```python
from build123d import *

# Parameters (mm, degrees)
F0_W         = 20
F0_H         = 20
F1_DEPTH     = 20.8070650697
F3_DEPTH     = 10
F4_T4_DEPTH  = 23.6433897602
F4_T10_DEPTH = 23.6433897602
F4_T15_DEPTH = 23.6433897602
F4_T20_DEPTH = 23.6433897602
F4_T26_DEPTH = 23.6433897602
F4_T32_DEPTH = 23.6433897602
F4_T39_DEPTH = 23.6433897602
F4_T44_DEPTH = 23.6433897602
F4_T52_DEPTH = 23.6433897602
F4_T57_DEPTH = 23.6433897602
F4_T65_DEPTH = 23.6433897602
F4_T70_DEPTH = 23.6433897602


# Not quite as in the source:
# - a fillet or chamfer that OpenCascade refuses, or shapes differently, is made with other operations: its cross-section is extruded or revolved along the edge and cut away or added


with BuildPart() as f1:
    # F0 (on Front) → F1 (new body)
    with BuildSketch(Plane.XZ):
        with Locations((10, 10)):
            Rectangle(F0_W, F0_H)
    extrude(amount=F1_DEPTH)

    # F2 (on face) → F3 (cut)
    with BuildSketch(Plane.XY.offset(20)):
        Polygon((10, -18.2805472855), (16.8216948801, -6.4650251595), (3.1783051199, -6.4650251595), align=None)
    extrude(amount=-F3_DEPTH, mode=Mode.SUBTRACT)

    # F4: fillet of radius 2 on 6 edges, made by hand


with BuildPart() as f4_tool2:
    # F4_s3 → F4_t4 (new body)
    with BuildSketch(Plane.YZ.offset(21.8216948801)):
        with BuildLine():
            ThreePointArc((-6.4650251595, 12), (-7.0508115971, 10.5857864376), (-8.4650251595, 10))
            Line((-8.4650251595, 10), (-6.4650251595, 10))
            Line((-6.4650251595, 10), (-6.4650251595, 12))
        make_face()
    extrude(amount=-F4_T4_DEPTH)

    split(bisect_by=Plane(origin=(-0.4157091722, -0.2400098025, 0), x_dir=(0, 0, 1), z_dir=(0.8660254038, 0.5, 0)), keep=Keep.TOP)

    split(bisect_by=Plane(origin=(15.4157091722, -8.9002638403, 0), x_dir=(0, 0, 1), z_dir=(-0.8660254038, 0.5, 0)), keep=Keep.TOP)


with BuildPart() as f1_1:
    add(f1.part)

    # F4_t1: union F4_tool2
    add(f4_tool2.part)


with BuildPart() as f4_tool8:
    # F4_s9 → F4_t10 (new body)
    with BuildSketch(Plane(origin=(-7.9157091722, -13.7104104641, 0), x_dir=(0, 0, 1), z_dir=(0.5, 0.8660254038, 0))):
        with BuildLine():
            ThreePointArc((12, 17.8005276806), (10.5857864376, 17.214741243), (10, 15.8005276806))
            Line((10, 15.8005276806), (10, 17.8005276806))
            Line((10, 17.8005276806), (12, 17.8005276806))
        make_face()
    extrude(amount=F4_T10_DEPTH)

    split(bisect_by=Plane(origin=(-0.4157091722, -0.2400098025, 0), x_dir=(0, 0, 1), z_dir=(0.8660254038, 0.5, 0)), keep=Keep.TOP)


with BuildPart() as f1_2:
    add(f1_1.part)

    # F4_t7: union F4_tool8
    add(f4_tool8.part)


with BuildPart() as f4_tool13:
    # F4_s14 → F4_t15 (new body)
    with BuildSketch(Plane(origin=(1.0940142921, -1.8948883381, 0), x_dir=(0, 0, 1), z_dir=(0.5, -0.8660254038, 0))):
        with BuildLine():
            ThreePointArc((12, 0.4800196049), (10.5857864376, -0.1057668327), (10, -1.5199803951))
            Line((10, -1.5199803951), (10, 0.4800196049))
            Line((10, 0.4800196049), (12, 0.4800196049))
        make_face()
    extrude(amount=F4_T15_DEPTH)

    split(bisect_by=Plane(origin=(15.4157091722, -8.9002638403, 0), x_dir=(0, 0, 1), z_dir=(-0.8660254038, 0.5, 0)), keep=Keep.TOP)


with BuildPart() as f1_3:
    add(f1_2.part)

    # F4_t12: union F4_tool13
    add(f4_tool13.part)


with BuildPart() as f4_tool18:
    # F4_s19 → F4_t20 (new body)
    with BuildSketch(Plane(origin=(-7.9157091722, -13.7104104641, 0), x_dir=(0, 0, 1), z_dir=(0.5, 0.8660254038, 0))):
        with BuildLine():
            ThreePointArc((20, 19.8005276806), (19.4142135624, 18.3863141182), (18, 17.8005276806))
            Line((18, 17.8005276806), (20, 17.8005276806))
            Line((20, 17.8005276806), (20, 19.8005276806))
        make_face()
    extrude(amount=F4_T20_DEPTH)

    split(bisect_by=Plane(origin=(-0.4157091722, -0.2400098025, 0), x_dir=(0, 0, 1), z_dir=(0.8660254038, 0.5, 0)), keep=Keep.TOP)

    split(bisect_by=Plane.XZ.offset(6.4650251595), keep=Keep.TOP)


with BuildPart() as f1_4:
    add(f1_3.part)

    # F4_t17: cut F4_tool18
    add(f4_tool18.part, mode=Mode.SUBTRACT)


with BuildPart() as f4_tool24:
    # F4_s25 → F4_t26 (new body)
    with BuildSketch(Plane(origin=(1.0940142921, -1.8948883381, 0), x_dir=(0, 0, 1), z_dir=(0.5, -0.8660254038, 0))):
        with BuildLine():
            ThreePointArc((20, 2.4800196049), (19.4142135624, 1.0658060425), (18, 0.4800196049))
            Line((18, 0.4800196049), (20, 0.4800196049))
            Line((20, 0.4800196049), (20, 2.4800196049))
        make_face()
    extrude(amount=F4_T26_DEPTH)

    split(bisect_by=Plane.XZ.offset(6.4650251595), keep=Keep.TOP)

    split(bisect_by=Plane(origin=(15.4157091722, -8.9002638403, 0), x_dir=(0, 0, 1), z_dir=(-0.8660254038, 0.5, 0)), keep=Keep.TOP)


with BuildPart() as f1_5:
    add(f1_4.part)

    # F4_t23: cut F4_tool24
    add(f4_tool24.part, mode=Mode.SUBTRACT)


with BuildPart() as f4_tool30:
    # F4_s31 → F4_t32 (new body)
    with BuildSketch(Plane.YZ.offset(21.8216948801)):
        with BuildLine():
            ThreePointArc((-4.4650251595, 20), (-5.8792387219, 19.4142135624), (-6.4650251595, 18))
            Line((-6.4650251595, 18), (-6.4650251595, 20))
            Line((-6.4650251595, 20), (-4.4650251595, 20))
        make_face()
    extrude(amount=-F4_T32_DEPTH)

    split(bisect_by=Plane(origin=(-0.4157091722, -0.2400098025, 0), x_dir=(0, 0, 1), z_dir=(0.8660254038, 0.5, 0)), keep=Keep.TOP)

    split(bisect_by=Plane(origin=(15.4157091722, -8.9002638403, 0), x_dir=(0, 0, 1), z_dir=(-0.8660254038, 0.5, 0)), keep=Keep.TOP)


with BuildPart() as f1_6:
    add(f1_5.part)

    # F4_t29: cut F4_tool30
    add(f4_tool30.part, mode=Mode.SUBTRACT)


with BuildPart() as f4_tool37:
    # F4_s38 → F4_t39 (new body)
    with BuildSketch(Plane(origin=(1.0940142921, -1.8948883381, 0), x_dir=(0, 0, 1), z_dir=(0.5, -0.8660254038, 0))):
        with BuildLine():
            ThreePointArc((20, 2.4800196049), (19.4142135624, 1.0658060425), (18, 0.4800196049))
            Line((18, 0.4800196049), (20, 0.4800196049))
            Line((20, 0.4800196049), (20, 2.4800196049))
        make_face()
    extrude(amount=F4_T39_DEPTH)

    split(bisect_by=Plane.XZ.offset(20.8070650697), keep=Keep.BOTTOM)

    split(bisect_by=Plane(origin=(15.4157091722, -8.9002638403, 0), x_dir=(0, 0, 1), z_dir=(0.8660254038, -0.5, 0)), keep=Keep.TOP)


with BuildPart() as f4_tool42:
    # F4_s43 → F4_t44 (new body)
    with BuildSketch(Plane(origin=(-7.9157091722, -13.7104104641, 0), x_dir=(0, 0, 1), z_dir=(0.5, 0.8660254038, 0))):
        with BuildLine():
            ThreePointArc((20, 19.8005276806), (19.4142135624, 18.3863141182), (18, 17.8005276806))
            Line((18, 17.8005276806), (20, 17.8005276806))
            Line((20, 17.8005276806), (20, 19.8005276806))
        make_face()
    extrude(amount=F4_T44_DEPTH)

    split(bisect_by=Plane.XZ.offset(20.8070650697), keep=Keep.BOTTOM)

    split(bisect_by=Plane(origin=(-0.4157091722, -0.2400098025, 0), x_dir=(0, 0, 1), z_dir=(-0.8660254038, -0.5, 0)), keep=Keep.TOP)


with BuildPart() as f4_tool37_1:
    add(f4_tool37.part)

    # F4_t47: intersect F4_tool42
    add(f4_tool42.part, mode=Mode.INTERSECT)


with BuildPart() as f1_7:
    add(f1_6.part)

    # F4_t35: cut F4_tool37
    add(f4_tool37_1.part, mode=Mode.SUBTRACT)


with BuildPart() as f4_tool50:
    # F4_s51 → F4_t52 (new body)
    with BuildSketch(Plane.YZ.offset(21.8216948801)):
        with BuildLine():
            ThreePointArc((-4.4650251595, 20), (-5.8792387219, 19.4142135624), (-6.4650251595, 18))
            Line((-6.4650251595, 18), (-6.4650251595, 20))
            Line((-6.4650251595, 20), (-4.4650251595, 20))
        make_face()
    extrude(amount=-F4_T52_DEPTH)

    split(bisect_by=Plane.YZ.offset(20), keep=Keep.BOTTOM)

    split(bisect_by=Plane(origin=(15.4157091722, -8.9002638403, 0), x_dir=(0, 0, 1), z_dir=(0.8660254038, -0.5, 0)), keep=Keep.TOP)


with BuildPart() as f4_tool55:
    # F4_s56 → F4_t57 (new body)
    with BuildSketch(Plane(origin=(-7.9157091722, -13.7104104641, 0), x_dir=(0, 0, 1), z_dir=(0.5, 0.8660254038, 0))):
        with BuildLine():
            ThreePointArc((20, 19.8005276806), (19.4142135624, 18.3863141182), (18, 17.8005276806))
            Line((18, 17.8005276806), (20, 17.8005276806))
            Line((20, 17.8005276806), (20, 19.8005276806))
        make_face()
    extrude(amount=F4_T57_DEPTH)

    split(bisect_by=Plane.YZ.offset(20), keep=Keep.BOTTOM)

    split(bisect_by=Plane.XZ.offset(6.4650251595), keep=Keep.BOTTOM)


with BuildPart() as f4_tool50_1:
    add(f4_tool50.part)

    # F4_t60: intersect F4_tool55
    add(f4_tool55.part, mode=Mode.INTERSECT)


with BuildPart() as f1_8:
    add(f1_7.part)

    # F4_t48: cut F4_tool50
    add(f4_tool50_1.part, mode=Mode.SUBTRACT)


with BuildPart() as f4_tool63:
    # F4_s64 → F4_t65 (new body)
    with BuildSketch(Plane(origin=(1.0940142921, -1.8948883381, 0), x_dir=(0, 0, 1), z_dir=(0.5, -0.8660254038, 0))):
        with BuildLine():
            ThreePointArc((20, 2.4800196049), (19.4142135624, 1.0658060425), (18, 0.4800196049))
            Line((18, 0.4800196049), (20, 0.4800196049))
            Line((20, 0.4800196049), (20, 2.4800196049))
        make_face()
    extrude(amount=F4_T65_DEPTH)

    split(bisect_by=Plane.YZ, keep=Keep.TOP)

    split(bisect_by=Plane.XZ.offset(6.4650251595), keep=Keep.BOTTOM)


with BuildPart() as f4_tool68:
    # F4_s69 → F4_t70 (new body)
    with BuildSketch(Plane.YZ.offset(21.8216948801)):
        with BuildLine():
            ThreePointArc((-4.4650251595, 20), (-5.8792387219, 19.4142135624), (-6.4650251595, 18))
            Line((-6.4650251595, 18), (-6.4650251595, 20))
            Line((-6.4650251595, 20), (-4.4650251595, 20))
        make_face()
    extrude(amount=-F4_T70_DEPTH)

    split(bisect_by=Plane.YZ, keep=Keep.TOP)

    split(bisect_by=Plane(origin=(-0.4157091722, -0.2400098025, 0), x_dir=(0, 0, 1), z_dir=(-0.8660254038, -0.5, 0)), keep=Keep.TOP)


with BuildPart() as f4_tool63_1:
    add(f4_tool63.part)

    # F4_t73: intersect F4_tool68
    add(f4_tool68.part, mode=Mode.INTERSECT)


with BuildPart() as f1_9:
    add(f1_8.part)

    # F4_t61: cut F4_tool63
    add(f4_tool63_1.part, mode=Mode.SUBTRACT)


solid = f1_9.part
```
Can you work these out from the model? Positions are in its coordinate system, mm. A direction names the side the tool comes from. Coordinates: 2 decimals unless noted, no trailing zeros. Write each loop counter-clockwise with the first axis right and the second up, starting at its lowest first coordinate (ties: lowest second). Pieces come first, ordered by that corner, then holes. Notation, with made-up numbers: M 76,81 L 94,81 A23 ccw 94,90 Z; hole C 79,8.5 d6. An arc over 180 degrees is marked long. Write item = value, one per line. Start each with the question number.
Q1. If I drill on L1, parallel to X at y = -17.75, z = 13.75; L2, parallel to X at y = -16, z = 12; L3, parallel to Y at x = 8, z = 13.5, over which ranges is the centre line in solid material (lowest first)? Write a range as [from, to].
Q2. If we section it at B-B, the plane z = 11: Write out the boundary of the cut face in (x, y).
Q3. I'm going to push a flat-ended pin straight in: pin 1 (1.7 mm diameter, centred on x = 11.5, y = -12, fed in from +Z). Where does the tip first touch, or does it pass through?
Q4. Thinking about a two-plate mould opening in X: for faces 1 (the face through (10, -20.807, 10)), 2 (the face through (20, -10, 10)), 3 (the face through (6.844, -12.115, 10.871)), which applies, released by +X, released by -X, zero draft, split by the parting line, or undercut?
Q5. If we section it at A-A, the plane z = 16.75: Write out the boundary of the cut face in (x, y).
Q6. On a 3-axis mill with a long thin cutter (end or side, diameter ignored), from which of +Z, -Z, +X, -X, +Y, -Y can I reach the whole of each face in a straight line? I mean faces 4 (the face through (10, -11, 10)), 5 (the face through (10, 0, 10)). Say none if no direction works.
Check sheet entries:
q1.L1 = [0, 9.69], [10.31, 20]
q1.L2 = [0, 8.68], [11.32, 20]
q1.L3 = [-20.81, -14.82], [-6.47, 0]
q2.outline = M 0,-20.81 L 20,-20.81 L 20,0 L 0,0 Z; hole M 3.64,-6.73 L 10,-17.74 L 16.36,-6.73 Z
q3.pin_1 = 10.27
q4.face_1 = zero draft
q4.face_2 = released by +X
q4.face_3 = undercut
q5.outline = M 0,-20.81 L 20,-20.81 L 20,0 L 0,0 Z; hole M 3.18,-6.47 L 10,-18.28 L 16.82,-6.47 Z
q6.face_4 = +Z
q6.face_5 = +Z, -Z, +X, -X, +Y
